from build123d import *

# Parameters (mm, degrees)
F0_W     = 2381.25
F0_H     = 28.575
F1_DEPTH = 698.5
F3_W     = 0.762
F3_H     = 698.5
F3_W_2   = 28.575
F3_W_3   = 726.313
F4_DEPTH = 28.575
F2_W     = 726.313
F2_H     = 698.5
F2_W_2   = 28.575
F2_W_3   = 0.762
F5_DEPTH = 28.575


with BuildPart() as f1:
    # F0 (on Top) → F1 (new body)
    with BuildSketch(Plane.XY):
        with Locations((933.8365292177, 70.3620000839)):
            Rectangle(F0_W, F0_H)
    extrude(amount=F1_DEPTH)

    # F3 (on face) → F4 (join)
    with BuildSketch(Plane(origin=(-256.7884707823, 0, 0), x_dir=(0, -1, 0), z_dir=(-1, 0, 0))):
        with Locations((-85.0305000839, 349.25)):
            Rectangle(F3_W, F3_H)
        with Locations((-70.3620000839, 349.25)):
            Rectangle(F3_W_2, F3_H)
        with Locations((307.0819999161, 349.25)):
            Rectangle(F3_W_3, F3_H)
    extrude(amount=F4_DEPTH)

    # F2 (on face) → F5 (join)
    with BuildSketch(Plane.YZ.offset(2124.4615292177)):
        with Locations((-307.0819999161, 349.25)):
            Rectangle(F2_W, F2_H)
        with Locations((70.3620000839, 349.25)):
            Rectangle(F2_W_2, F2_H)
        with Locations((85.0305000839, 349.25)):
            Rectangle(F2_W_3, F2_H)
    extrude(amount=F5_DEPTH)


solid = f1.part
Could you check a few things on this model? Use its own coordinates, in mm. A direction names the side the tool comes from. Round coordinates to 2 decimals unless told otherwise and drop trailing zeros. Order: outer loops, then holes, each group sorted by start corner. A loop starts at its lowest first (then second) coordinate and runs counter-clockwise, first axis right, second up.
Q1. Which directions (+Z, -Z, +X, -X, +Y, -Y) give clear straight access to the entire face, cutting with the end or side of a thin tool? Please do faces 1 (the face through (-285.363, -287, 354)), 2 (the face through (-256.788, -302, 354)).
Geometry says:
face 1: +Z, -Z, -X, +Y, -Y
face 2: +Z, -Z, -Y
Q2. I'm going to push flat-ended pins straight in: P1, Ø12, axis at x = 502.5, z = 354.5, coming from the +Y side; P2, Ø1.5, axis at x = 421.5, z = 483.5, coming from the -Y side. Where does each tip first touch, or does it pass through?
Geometry says:
P1: stops at y = 84.65
P2: stops at y = 56.07
Q3. Imagine slicing it at B-B, the plane z = 358.5. List the corners of the cut face in (x, y) for me, then the cut area to 3 significant figures.
Geometry says:
outline: (-285.36, -670.24) - (-256.79, -670.24) - (-256.79, 56.07) - (2124.46, 56.07) - (2124.46, -670.24) - (2153.04, -670.24) - (2153.04, 85.41) - (2124.46, 85.41) - (2124.46, 84.65) - (-256.79, 84.65) - (-256.79, 85.41) - (-285.36, 85.41) - close
area: 111,000 mm2
Q4. Thinking about a two-plate mould opening in X: for faces 3 (the face through (2124.462, -312, 354)), 4 (the face through (2153.037, -298, 354)), 5 (the face through (928, 70, 0)), which applies, released by +X, released by -X, zero draft, split by the parting line, or undercut?
Geometry says:
face 3: undercut
face 4: released by +X
face 5: zero draft
Q5. Imagine slicing it at A-A, the plane y = -381.5. List the corners of the cut face in (x, z) for me.
Geometry says:
outline: (-285.36, 0) - (-256.79, 0) - (-256.79, 698.5) - (-285.36, 698.5) - close; (2124.46, 0) - (2153.04, 0) - (2153.04, 698.5) - (2124.46, 698.5) - close
Q6. Please list where these lines run through material, in increasing order: probe 1 along X at (y, z) = (-170, 174); probe 2 along Y at (x, z) = (-170, 90.5).
Geometry says:
probe 1: x = -285.36 to -256.79, 2124.46 to 2153.04
probe 2: y = 56.07 to 84.65
Q7. Imagine slicing it at C-C, the plane x = 1286.5. List the corners of the cut face in (y, z) for me.
Geometry says:
outline: (56.07, 0) - (84.65, 0) - (84.65, 698.5) - (56.07, 698.5) - close
